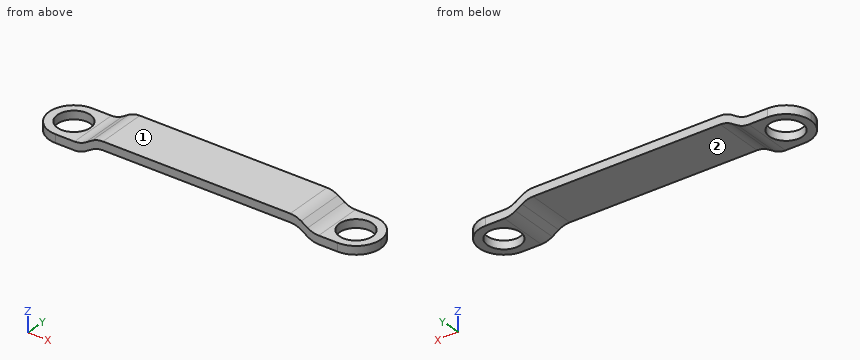
```python
from build123d import *

# Parameters (mm, degrees)
F2_DEPTH = 3.81
F3_D     = 5.08
F3_DEPTH = 3.81
F3_TIP   = 1.5261859723
F4_R     = 3.80999


# Not quite as in the source:
# - a fillet or chamfer is up to 0.001 mm smaller than in the source, because OpenCascade refuses the exact size


with BuildPart() as f2:
    # F1 (on Front) → F2 (new body, symmetric)
    with BuildSketch(Plane.XZ):
        with BuildLine():
            Line((-25.4, 1.27), (-25.4, 0))
            Line((-25.4, 0), (-18.6905780189, 0))
            ThreePointArc((-18.6905780189, 0), (-17.8152860399, 0.1230352309), (-17.0078313843, 0.4826053848))
            Line((-17.0078313843, 0.4826053848), (-16.0121686157, 1.1048946152))
            ThreePointArc((-16.0121686157, 1.1048946152), (-15.2047139601, 1.4644647691), (-14.3294219811, 1.5875))
            Line((-14.3294219811, 1.5875), (14.3294219811, 1.5875))
            ThreePointArc((14.3294219811, 1.5875), (15.2047139601, 1.4644647691), (16.0121686157, 1.1048946152))
            Line((16.0121686157, 1.1048946152), (17.0078313843, 0.4826053848))
            ThreePointArc((17.0078313843, 0.4826053848), (17.8152860399, 0.1230352309), (18.6905780189, 0))
            Line((18.6905780189, 0), (25.4, 0))
            Line((25.4, 0), (25.4, 1.27))
            Line((25.4, 1.27), (18.6905780189, 1.27))
            ThreePointArc((18.6905780189, 1.27), (17.8152860399, 1.3930352309), (17.0078313843, 1.7526053848))
            Line((17.0078313843, 1.7526053848), (16.0121686157, 2.3748946152))
            ThreePointArc((16.0121686157, 2.3748946152), (15.2047139601, 2.7344647691), (14.3294219811, 2.8575))
            Line((14.3294219811, 2.8575), (-14.3294219811, 2.8575))
            ThreePointArc((-14.3294219811, 2.8575), (-15.2047139601, 2.7344647691), (-16.0121686157, 2.3748946152))
            Line((-16.0121686157, 2.3748946152), (-17.0078313843, 1.7526053848))
            ThreePointArc((-17.0078313843, 1.7526053848), (-17.8152860399, 1.3930352309), (-18.6905780189, 1.27))
            Line((-18.6905780189, 1.27), (-25.4, 1.27))
        make_face()
    extrude(amount=F2_DEPTH, both=True)

    # F3
    with Locations(Plane(origin=(0, 0, 0), x_dir=(1, 0, 0), z_dir=(0, 0, -1))):
        with Locations((-21.59, 0), (21.59, 0)):
            Hole(F3_D / 2, depth=F3_DEPTH)
            with Locations((0, 0, -(F3_DEPTH + F3_TIP / 2))):  # 118° drill point
                Cone(0, F3_D / 2, F3_TIP, mode=Mode.SUBTRACT)

    # F4 (radius 3.81 in the source; OpenCascade refuses exactly that, so slightly less here)
    f4_edges = [f2.edges().sort_by_distance(p)[0] for p in [
        (-25.4, -3.81, 0.635),
        (-25.4, 3.81, 0.635),
        (25.4, -3.81, 0.635),
        (25.4, 3.81, 0.635),
    ]]
    fillet(f4_edges, radius=F4_R)


solid = f2.part
```
Check sheet for the modelled part. Datum: model origin and axes. Units: mm. Face numbers are marked on the shaded views. Give positions to 0.01 mm unless a question says otherwise; leave off trailing zeros. Order: outer loops, then holes, each group sorted by start corner. A loop starts at its lowest first (then second) coordinate and runs counter-clockwise, first axis right, second up. Notation, with made-up numbers: M -3,78 L 40,78 A8 ccw 40,82 Z; hole C 89.25,28 d3. An arc over 180 degrees is marked long. Answer in a Markdown table with one row per item.
1) Cross-section at B-B, the plane x = -13.5. Enter the section's corners in (y, z).
Filled sheet:
| item | result |
|---|---|
| outline | M -3.81,1.59 L 3.81,1.59 L 3.81,2.86 L -3.81,2.86 Z |
2) Gauge pin test, flat end, axial feed: P1, Ø1, axis at y = 1.5, z = 2, coming from the -X side. Record the tip position at first contact, or that the pin passes through.
Filled sheet:
| item | result |
|---|---|
| P1 | stops at x = -17.5 |
3) Thickness scan on L1, parallel to Y at x = -21.59, z = 0.8; L2, parallel to Z at x = -14.5, y = -0.25; L3, parallel to X at y = -0.25, z = 0.7. Record the ranges inside material, lowest first. Write a range as [from, to].
Filled sheet:
| item | result |
|---|---|
| L1 | y = [-3.81, -2.54], [2.54, 3.81] |
| L2 | z = [1.58, 2.85] |
| L3 | x = [-25.39, -24.12], [-19.06, -16.66], [16.66, 19.06], [24.12, 25.39] |
4) Release check for a two-part mould opening along X. For the marked faces 1 and 2 record: +X half, -X half, draft (parallel to the pull), parting line (faces both ways), or undercut.
Filled sheet:
| item | result |
|---|---|
| face 1 | draft |
| face 2 | undercut |
